Here's the drawing with two shaded views (mm, measured from the low corner). I have some questions. Give positions to 0.01 mm unless a question says otherwise; leave off trailing zeros. Loops run counter-clockwise (first coordinate to the right, second up) from the corner with the lowest first, then second, coordinate; pieces in that order, holes last. Notation, with made-up numbers: M 33.25,3 L 39.25,3 A32 ccw 39.25,42 Z; hole C 69,-22.75 d11. An arc over 180 degrees is marked long. Use CSV: the item, a comma, the result in double quotes.
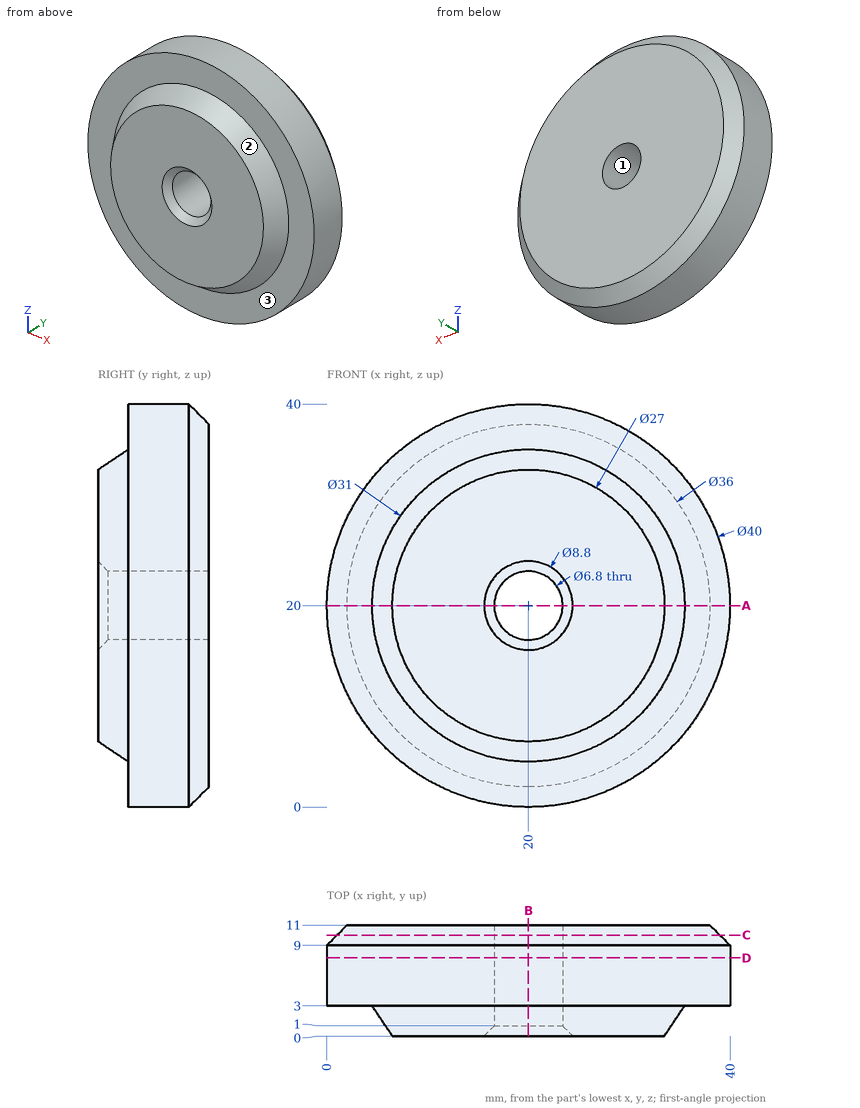
1. I want a section at C-C, the plane y = 10. List the corners of the cut face in (x, z) for me, then the cut area to 3 significant figures.
Outcome:
outline,"C 20,20 d38; hole C 20,20 d6.8"
area,"1,100 mm2"
2. I want a section at A-A, the plane z = 20. List the corners of the cut face in (x, y) for me.
Outcome:
outline,"M 0,3 L 4.5,3 L 6.5,0 L 15.6,0 L 16.6,1 L 16.6,11 L 2,11 L 0,9 Z; M 23.4,1 L 24.4,0 L 33.5,0 L 35.5,3 L 40,3 L 40,9 L 38,11 L 23.4,11 Z"
3. I want a section at B-B, the plane x = 20. List the corners of the cut face in (y, z) for me, then the cut area to 3 significant figures.
Outcome:
outline,"M 0,6.5 L 3,4.5 L 3,0 L 9,0 L 11,2 L 11,16.6 L 1,16.6 L 0,15.6 Z; M 0,24.4 L 1,23.4 L 11,23.4 L 11,38 L 9,40 L 3,40 L 3,35.5 L 0,33.5 Z"
area,"327 mm2"
4. I want a section at D-D, the plane y = 7.75. List the corners of the cut face in (x, z) for me.
Outcome:
outline,"C 20,20 d40; hole C 20,20 d6.8"
5. I'm going to push flat-ended pins straight in: pin 1 Ø6 at (y, z) = (8.5, 13.5) entering from +X; pin 2 Ø2 at (x, y) = (36, 4) entering from +Z; pin 3 Ø1 at (x, y) = (27.5, 8) entering from -Z (3 decimals). Where does each tip first touch, or does it pass through?
Outcome:
pin 1,"x = 39.69"
pin 2,"z = 33.23"
pin 3,"z = 1.265"
6. If we mould it in two halves opening along X, with no side actions, what happens to the marked faces 1, 2 and 3? For each: +X half, -X half, draft (parallel to the pull), parting line (faces both ways), or undercut.
Outcome:
face 1,"undercut"
face 2,"parting line"
face 3,"draft"
7. Please list where these lines run through material, in increasing order: line 1 (X direction, y = 3.5, z = 20); line 2 (Y direction, x = 32, z = 7.5); line 3 (Z direction, x = 18.5, y = 9.5).
Outcome:
line 1,"0 to 16.6, 23.4 to 40"
line 2,"3 to 11"
line 3,"0.56 to 16.95, 23.05 to 39.44"
